The listing builds one solid part. Answer for the finished solid, in the listing's coordinates (mm). A direction names the side the tool comes from. Give positions to 0.01 mm unless a question says otherwise; leave off trailing zeros. Loops run counter-clockwise (first coordinate to the right, second up) from the corner with the lowest first, then second, coordinate; pieces in that order, holes last.
Item 1: Section A-A, the plane z = -7 is taken. Give the vertices of the cut face in (x, y), and give its area (3 significant figures).
Item 2: Consider line 1 along X through (y, z) = (3.5, -68); line 2 along Z through (x, y) = (31.5, 41). Determine where each line is inside the solid, lowest interval first.
Item 3: This flat-tipped pin is pushed along its axis until it touches: pin 1 Ø1 at (x, y) = (23, 44.5) entering from -Z. Where does it stop, or does it pass through?
Item 4: Section B-B, the plane y = 9.5 is taken. Give the vertices of the cut face in (x, z), and give its area (3 significant figures).
Item 5: The mould has two halves that part along Y. Classify faces 1 (the face through (23, 1, -90)), 2 (the face through (2, 25, -44)), 3 (the face through (25, 26, 0)), 4 (the face through (25, 50.8, -44)): pulls with the +Y half, pulls with the -Y half, needs draft (parallel to the pull), parting line crosses it, or undercut.
Item 6: A tool of negligible diameter and unlimited length cuts with its end or side. For faces 5 (the face through (25, 0, -44)), 6 (the face through (25, 2, -44)), from which of +Z, -Z, +X, -X, +Y, -Y can it reach the whole face along a straight path? Write none if from no direction.
from build123d import *

# Parameters (mm, degrees)
SKETCH1_W           = 50.8
SKETCH1_H           = 50.8
SKETCH1_W_2         = 46.8
SKETCH1_H_2         = 46.8
BOSS_EXTRUDE1_DEPTH = 1
SKETCH1_3_W         = 50.8
SKETCH1_3_H         = 50.8
SKETCH1_3_W_2       = 46.8
SKETCH1_3_H_2       = 46.8
BOSS_EXTRUDE2_DEPTH = 90
FILLET1_R           = 1


with BuildPart() as part:
    # Sketch1 → Boss-Extrude1 (new body)
    with BuildSketch(Plane.XY):
        with Locations((25.4, 25.4)):
            Rectangle(SKETCH1_W, SKETCH1_H)
        with Locations((25.4, 25.4)):
            Rectangle(SKETCH1_W_2, SKETCH1_H_2, mode=Mode.SUBTRACT)
        with Locations((25.4, 25.4)):
            Rectangle(SKETCH1_W_2, SKETCH1_H_2)
    extrude(amount=BOSS_EXTRUDE1_DEPTH)

    # Sketch1_3 → Boss-Extrude2 (add)
    with BuildSketch(Plane.XY):
        with Locations((25.4, 25.4)):
            Rectangle(SKETCH1_3_W, SKETCH1_3_H)
        with Locations((25.4, 25.4)):
            Rectangle(SKETCH1_3_W_2, SKETCH1_3_H_2, mode=Mode.SUBTRACT)
    extrude(amount=-BOSS_EXTRUDE2_DEPTH)

    # Fillet1
    fillet1_edges = [part.edges().sort_by_distance(p)[0] for p in [
        (0, 0, -44.5),
        (0, 50.8, -44.5),
        (50.8, 50.8, -44.5),
        (50.8, 0, -44.5),
    ]]
    fillet(fillet1_edges, radius=FILLET1_R)


solid = part.part
Worked answers:
1. outline: (0, 1) arc R1 ccw to (1, 0) - (49.8, 0) arc R1 ccw to (50.8, 1) - (50.8, 49.8) arc R1 ccw to (49.8, 50.8) - (1, 50.8) arc R1 ccw to (0, 49.8) - close; hole (2, 2) - (48.8, 2) - (48.8, 48.8) - (2, 48.8) - close
1. area: 390 mm2
2. line 1: x = 0 to 2, 48.8 to 50.8
2. line 2: z = 0 to 1
3. pin 1: stops at z = 0
4. outline: (0, -90) - (2, -90) - (2, 0) - (48.8, 0) - (48.8, -90) - (50.8, -90) - (50.8, 1) - (0, 1) - close
4. area: 411 mm2
5. face 1: needs draft
5. face 2: undercut
5. face 3: undercut
5. face 4: pulls with the +Y half
6. face 5: +Z, -Z, +X, -X, -Y
6. face 6: -Z
